Can you work these out from the model? Positions are in its coordinate system, mm. Coordinates: 2 decimals unless noted, no trailing zeros. Order: outer loops, then holes, each group sorted by start corner. A loop starts at its lowest first (then second) coordinate and runs counter-clockwise, first axis right, second up. Notation, with made-up numbers: (-23.75, 30.5) -> (3.25, 30.5) arc R9 cw to (3.25, 44.5) -> close; hole circle Ø10 at (-31, -24). An arc over 180 degrees is marked (long way). Answer in a Markdown table with one row per item.
```python
from build123d import *

# Parameters (mm, degrees)
SKETCH1_R                = 1.651
BOSS_EXTRUDE2_DEPTH      = 3.048
SKETCH5_W                = 36.105919561
SKETCH5_H                = 30.801250688
SKETCH5_W_2              = 35.958513686
SKETCH5_H_2              = 33.469345806
BOSS_EXTRUDE4_DEPTH      = 3.048
SKETCH11_R               = 1.651
CUT_EXTRUDE7_DEPTH       = 106.247375758
BOSS_EXTRUDE6_DEPTH      = 3.048
SKETCH14_W               = 25.4
SKETCH14_H               = 69.85
CUT_EXTRUDE9_DEPTH       = 46.482
SKETCH15_R               = 1.651
CUT_EXTRUDE10_DEPTH      = 150.876
SKETCH16_R               = 1.5
CUT_EXTRUDE11_DEPTH      = 107.010848992
SKETCH17_R               = 3.175
CUT_EXTRUDE12_DEPTH      = 103.378
CUT_EXTRUDE12_DEPTH_BACK = 48.768


with BuildPart() as part:
    # Sketch1 → Boss-Extrude2 (new body)
    with BuildSketch(Plane.XY):
        with BuildLine():
            Line((-73.845886141, 12.7), (-56.065886141, 12.7))
            Line((-56.065886141, 12.7), (-56.065886141, -12.7))
            Line((-56.065886141, -12.7), (-73.845886141, -12.7))
            ThreePointArc((-73.845886141, -12.7), (0, -74.93), (73.845886141, -12.7))
            Line((73.845886141, -12.7), (56.065886141, -12.7))
            Line((56.065886141, -12.7), (56.065886141, 12.7))
            Line((56.065886141, 12.7), (73.845886141, 12.7))
            ThreePointArc((73.845886141, 12.7), (0, 74.93), (-73.845886141, 12.7))
        make_face()
        with Locations(Location((-45.466, 11.049, 0), (0, 0, 180))):
            Circle(SKETCH1_R, mode=Mode.SUBTRACT)
        with Locations(Location((-20.067270032, 10.795, 0), (0, 0, 180))):
            Circle(SKETCH1_R, mode=Mode.SUBTRACT)
        with Locations(Location((-20.067270032, -10.795, 0), (0, 0, 180))):
            Circle(SKETCH1_R, mode=Mode.SUBTRACT)
        with Locations(Location((-45.466, -11.049, 0), (0, 0, 180))):
            Circle(SKETCH1_R, mode=Mode.SUBTRACT)
        with Locations(Location((45.466, -11.049, 0), (0, 0, 180))):
            Circle(SKETCH1_R, mode=Mode.SUBTRACT)
        with Locations(Location((20.067270032, -10.795, 0), (0, 0, 180))):
            Circle(SKETCH1_R, mode=Mode.SUBTRACT)
        with Locations(Location((20.067270032, 10.795, 0), (0, 0, 180))):
            Circle(SKETCH1_R, mode=Mode.SUBTRACT)
        with Locations(Location((45.466, 11.049, 0), (0, 0, 180))):
            Circle(SKETCH1_R, mode=Mode.SUBTRACT)
    extrude(amount=BOSS_EXTRUDE2_DEPTH)

    # Sketch5 → Boss-Extrude4 (add)
    with BuildSketch(Plane(origin=(0, 0, 0), x_dir=(-1, 0, 0), z_dir=(0, 0, -1))):
        with Locations((34.78484389, -0.38515144)):
            Rectangle(SKETCH5_W, SKETCH5_H)
        with Locations((-32.830563904, 0.948896119)):
            Rectangle(SKETCH5_W_2, SKETCH5_H_2)
    extrude(amount=-BOSS_EXTRUDE4_DEPTH)

    # Sketch11 → Cut-Extrude7 (cut, through all)
    with BuildSketch(Plane(origin=(0, 0, 0), x_dir=(-1, 0, 0), z_dir=(0, 0, -1))):
        with Locations((43.18, 53.975)):
            Circle(SKETCH11_R)
        with Locations((0, 53.975)):
            Circle(SKETCH11_R)
        with Locations((0, -14.605)):
            Circle(SKETCH11_R)
        with Locations((43.18, -14.605)):
            Circle(SKETCH11_R)
        with Locations((-43.18, 53.975)):
            Circle(SKETCH11_R)
        with Locations((-43.18, -14.605)):
            Circle(SKETCH11_R)
        with Locations((-25.4, -30.48)):
            Circle(SKETCH11_R)
        with Locations((-46.101, -43.8609994)):
            Circle(SKETCH11_R)
        with Locations((46.101, -43.8609994)):
            Circle(SKETCH11_R)
        with Locations((0, -64.77)):
            Circle(SKETCH11_R)
        with Locations((25.4, -30.48)):
            Circle(SKETCH11_R)
    extrude(amount=-CUT_EXTRUDE7_DEPTH, mode=Mode.SUBTRACT)

    # Sketch12 → Boss-Extrude6 (add)
    with BuildSketch(Plane(origin=(0, 0, 0), x_dir=(-1, 0, 0), z_dir=(0, 0, -1))):
        with BuildLine():
            Line((-54.995250635, 50.892310889), (-54.566459663, -51.351790425))
            ThreePointArc((-54.566459663, -51.351790425), (-74.929341077, -0.314238422), (-54.995250635, 50.892310889))
        make_face()
        with BuildLine():
            Line((54.995250635, 50.892310889), (54.995250635, -50.892310889))
            ThreePointArc((54.995250635, -50.892310889), (74.93, 0), (54.995250635, 50.892310889))
        make_face()
    extrude(amount=-BOSS_EXTRUDE6_DEPTH)

    # Sketch14 → Cut-Extrude9 (cut)
    with BuildSketch(Plane(origin=(0, 0, 0), x_dir=(-1, 0, 0), z_dir=(0, 0, -1))):
        with Locations((-20.32, 9.525)):
            Rectangle(SKETCH14_W, SKETCH14_H)
        with Locations((20.32, 9.525)):
            Rectangle(SKETCH14_W, SKETCH14_H)
    extrude(amount=-CUT_EXTRUDE9_DEPTH, mode=Mode.SUBTRACT)

    # Sketch15 → Cut-Extrude10 (cut)
    with BuildSketch(Plane(origin=(-30.092005081, 4.08352975, -68.453), x_dir=(-1, 0, 0), z_dir=(0, 0, -1))):
        with Locations(Location((-101.395980802, -12.71952975, 0), (0, 0, 180))):
            Circle(SKETCH15_R)
        with Locations(Location((-101.395980802, 4.55247025, 0), (0, 0, 180))):
            Circle(SKETCH15_R)
        with Locations(Location((41.211970641, -12.71952975, 0), (0, 0, 180))):
            Circle(SKETCH15_R)
        with Locations(Location((41.211970641, 4.55247025, 0), (0, 0, 180))):
            Circle(SKETCH15_R)
    extrude(amount=-CUT_EXTRUDE10_DEPTH, mode=Mode.SUBTRACT)

    # Sketch16 → Cut-Extrude11 (cut, through all)
    with BuildSketch(Plane(origin=(0, 0, 0), x_dir=(-1, 0, 0), z_dir=(0, 0, -1))):
        with Locations((-17.78, 66.04)):
            Circle(SKETCH16_R)
        with Locations((-57.15, 38.1)):
            Circle(SKETCH16_R)
        with Locations((17.78, 66.04)):
            Circle(SKETCH16_R)
        with Locations((-57.15, -38.1)):
            Circle(SKETCH16_R)
        with Locations((57.15, -38.1)):
            Circle(SKETCH16_R)
        with Locations((57.15, 38.1)):
            Circle(SKETCH16_R)
    extrude(amount=-CUT_EXTRUDE11_DEPTH, mode=Mode.SUBTRACT)

    # Sketch17 → Cut-Extrude12 (cut, two sides)
    with BuildSketch(Plane(origin=(-30.092005081, 4.08352975, -57.658), x_dir=(1, 0, 0), z_dir=(0, 0, 1))) as cut_extrude12_sk:
        with Locations((-16.897994919, 21.31647025)):
            Circle(SKETCH17_R)
        with Locations((77.082005081, 21.31647025)):
            Circle(SKETCH17_R)
        with Locations((30.092005081, 21.31647025)):
            Circle(SKETCH17_R)
        with Locations((77.082005081, -29.48352975)):
            Circle(SKETCH17_R)
        with Locations((30.092005081, -29.48352975)):
            Circle(SKETCH17_R)
        with Locations((-16.897994919, -29.48352975)):
            Circle(SKETCH17_R)
    extrude(amount=CUT_EXTRUDE12_DEPTH, mode=Mode.SUBTRACT)
    extrude(cut_extrude12_sk.sketch, amount=-CUT_EXTRUDE12_DEPTH_BACK, mode=Mode.SUBTRACT)


solid = part.part
```
(1) Suppose I cut it at B-B (y = 41.5). Please give me the cut outline in (x, z).
Response values:
| item | result |
|---|---|
| outline | (-62.39, 0) -> (-33.02, 0) -> (-33.02, 3.05) -> (-62.39, 3.05) -> close; (-7.62, 0) -> (7.62, 0) -> (7.62, 3.05) -> (-7.62, 3.05) -> close; (33.02, 0) -> (62.39, 0) -> (62.39, 3.05) -> (33.02, 3.05) -> close |
(2) Will these pins go through, and if not, where does the flat tip stop? pin 1 Ø3.5 at (x, y) = (-57.15, -38.1) entering from +Z; pin 2 Ø1.5 at (y, z) = (24.5, 2.5) entering from +X; pin 3 Ø1 at (x, z) = (-37, 1.5) entering from -Y.
Response values:
| item | result |
|---|---|
| pin 1 | z = 3.05 |
| pin 2 | x = 71.07 |
| pin 3 | y = -65.44 |
(3) We'd pull the mould along Y, two halves only. Please class faces 1 (the cylindrical face through (41.605, -14.109, 1.503)), 2 (the cylindrical face through (-47.626, -44.493, 1.503)), 3 (the flat face through (-1, 1, 3.048)): +Y half, -Y half, draft (parallel to the pull), parting line (faces both ways), or undercut.
Response values:
| item | result |
|---|---|
| face 1 | undercut |
| face 2 | undercut |
| face 3 | draft |
(4) Suppose I cut it at A-A (y = 4). Please give me the cut outline in (x, z).
Response values:
| item | result |
|---|---|
| outline | (-74.82, 0) -> (-33.02, 0) -> (-33.02, 3.05) -> (-74.82, 3.05) -> close; (-7.62, 0) -> (7.62, 0) -> (7.62, 3.05) -> (-7.62, 3.05) -> close; (33.02, 0) -> (74.82, 0) -> (74.82, 3.05) -> (33.02, 3.05) -> close |
(5) Suppose I cut it at C-C (z = 2.05). Count the separate pieces of the cut face and the enclosed holes in it, and give its area (3 significant figures).
Response values:
| item | result |
|---|---|
| separate pieces | 1 |
| enclosed holes | 29 |
| area | 13,700 mm2 |
(6) I need wall thicknesses on line 1 (Y direction, x = -27.5, z = 1.1); line 2 (Y direction, x = -43.18, z = 1.85); line 3 (X direction, y = -3.5, z = 2.95). Which ranges of each line are inside material? Lowest first, please. Write a range as [from, to].
Response values:
| item | result |
|---|---|
| line 1 | [-69.7, -25.4], [44.45, 69.7] |
| line 2 | [-61.24, -16.26], [-12.95, 52.32], [55.63, 61.24] |
| line 3 | [-74.85, -33.02], [-7.62, 7.62], [33.02, 74.85] |
(7) Suppose I cut it at D-D (y = -52). Please give me the cut outline in (x, z).
Response values:
| item | result |
|---|---|
| outline | (-53.95, 0) -> (53.95, 0) -> (53.95, 3.05) -> (-53.95, 3.05) -> close |
